Check sheet for the modelled part. Datum: model origin and axes. Units: mm. A direction names the side the tool comes from. Coordinates: 2 decimals unless noted, no trailing zeros. Write each loop counter-clockwise with the first axis right and the second up, starting at its lowest first coordinate (ties: lowest second). Pieces come first, ordered by that corner, then holes. Notation, with made-up numbers: (69, 71) -> (110, 71) arc R12 ccw to (110, 80) -> close; hole circle Ø9 at (79, 0.5). An arc over 180 degrees is marked (long way). One line per item, written item: value. Start each with the question number.
1) Gauge pin test, flat ends, axial feed: P1, Ø2, axis at x = 6.5, y = 8.5, coming from the +Z side; P2, Ø10, axis at x = 12.5, z = -29.5, coming from the -Y side. Record the tip position at first contact, or that the pin passes through.
2) Draft check along Z on faces 1 (the cylindrical face through (-16.76, -3.706, -43.397)), 2 (the cylindrical face through (16.74, 0.11, -37.815)), 3 (the cylindrical face through (-15.846, 12.629, -18.784)). Enter one of: +Z half, -Z half, draft (parallel to the pull), parting line (faces both ways), or undercut.
3) Sectioned sample at A-A on y = 0. Enter the section's corners in (x, z).
4) Sectioned sample at B-B on z = -39.5. Enter the section's corners in (x, y), plus the area to 3 significant figures.
5) Sectioned sample at D-D on x = -5.5. Enter the section's corners in (y, z).
6) Set-up check for faces 4 (the flat face through (-17.5, 4, -33)), 5 (the flat face through (-0.168, 12.845, -18.83)): record each of +Z, -Z, +X, -X, +Y, -Y from which the full face is reachable in a straight line by a thin tool's end or side.
7) Sectioned sample at C-C on z = -34.5. Enter the section's corners in (x, y).
8) Scan lines: line 1 along X through (y, z) = (13, -25); line 2 along Z through (x, y) = (-16.65, 0); line 3 along X through (y, z) = (17.25, -24). Record each from-to range of solid material in increasing order. Write a range as [from, to].
```python
from build123d import *

# Parameters (mm, degrees)
BOSS_EXTRUDE1_DEPTH            = 16
BOSS_EXTRUDE1_DEPTH_BACK       = 16
EDGE_FLANGE1_STRIP_W           = 14
EDGE_FLANGE1_STRIP_H           = 1.5
EDGE_FLANGE1_STRIP_CUT_DEPTH   = 15
EDGE_FLANGE1_STRIP_2_W         = 14
EDGE_FLANGE1_STRIP_2_H         = 1.5
EDGE_FLANGE1_STRIP_CUT_2_DEPTH = 15
EDGE_FLANGE1_DEPTH             = 15
EDGE_FLANGE1_BEND_DEPTH        = 15
CUT_EXTRUDE1_DEPTH             = 70.261521918
CUT_EXTRUDE1_DEPTH_BACK        = 70.261521918
SKETCH12_R                     = 2.5


# Sheet-metal steps are written as plain solids
with BuildPart() as part:
    # Sketch1 → Boss-Extrude1 (new, two sides: drawn at the far end of the back side and taken through both)
    with BuildSketch(Plane(origin=(0, 0, 0), x_dir=(0, 0, -1), z_dir=(1, 0, 0)).offset(-BOSS_EXTRUDE1_DEPTH_BACK)):
        Polygon((13.736581906, 7.002159097), (21.218242798, 20.003110997), (22.518337988, 19.254944908), (15.036677096, 6.253993008), align=None)
    extrude(amount=BOSS_EXTRUDE1_DEPTH + BOSS_EXTRUDE1_DEPTH_BACK)

    # Edge-Flange1 strip (across the edge) → Edge-Flange1 strip cut (cut)
    with BuildSketch(Plane(origin=(16, 19.254944908, -22.518337988), x_dir=(-1, 0, 0), z_dir=(0, -0.8667301266485011, 0.498777392791487))):
        with Locations((-3, -0.75)):
            Rectangle(EDGE_FLANGE1_STRIP_W, EDGE_FLANGE1_STRIP_H)
    extrude(amount=EDGE_FLANGE1_STRIP_CUT_DEPTH, mode=Mode.SUBTRACT)

    # Edge-Flange1 strip 2 (across the edge) → Edge-Flange1 strip cut 2 (cut)
    with BuildSketch(Plane(origin=(-16, 6.253993008, -15.036677096), x_dir=(1, 0, 0), z_dir=(0, 0.8667301266485011, -0.498777392791487))):
        with Locations((-3, -0.75)):
            Rectangle(EDGE_FLANGE1_STRIP_2_W, EDGE_FLANGE1_STRIP_2_H)
    extrude(amount=EDGE_FLANGE1_STRIP_CUT_2_DEPTH, mode=Mode.SUBTRACT)

    # Edge-Flange1 section (across the edge) → Edge-Flange1 (add)
    with BuildSketch(Plane(origin=(16, 19.254944908, -22.518337988), x_dir=(-1, 0, 0), z_dir=(0, -0.8667301266485011, 0.498777392791487))):
        with BuildLine():
            Line((-1.5, 4), (-1.5, 39))
            Line((-1.5, 39), (0, 39))
            Line((0, 39), (0, 4))
            ThreePointArc((0, 4), (1.171572875, 1.171572875), (4, 0))
            Line((4, 0), (4, -1.5))
            ThreePointArc((4, -1.5), (0.110912703, 0.110912703), (-1.5, 4))
        make_face()
    extrude(amount=EDGE_FLANGE1_DEPTH)

    # Edge-Flange1 section 2 (across the edge) → Edge-Flange1 bend (add)
    with BuildSketch(Plane(origin=(-16, 6.253993008, -15.036677096), x_dir=(1, 0, 0), z_dir=(0, 0.8667301266485011, -0.498777392791487))):
        with BuildLine():
            Line((-1.5, 4), (-1.5, 39))
            Line((-1.5, 39), (0, 39))
            Line((0, 39), (0, 4))
            ThreePointArc((0, 4), (1.171572875, 1.171572875), (4, 0))
            Line((4, 0), (4, -1.5))
            ThreePointArc((4, -1.5), (0.110912703, 0.110912703), (-1.5, 4))
        make_face()
    extrude(amount=EDGE_FLANGE1_BEND_DEPTH)

    # Sketch12 → Cut-Extrude1 (cut, two sides: drawn at the far end of the back side and taken through both)
    with BuildSketch(Plane(origin=(17.5, 0, 0), x_dir=(0, 0, -1), z_dir=(1, 0, 0)).offset(-CUT_EXTRUDE1_DEPTH_BACK)):
        with Locations((40.312429407, 0)):
            Circle(SKETCH12_R)
        with BuildLine():
            Line((33.525218207, -4.385612156), (48.839152035, -13.198325311))
            Line((48.839152035, -13.198325311), (56.320812927, -0.197373411))
            Line((56.320812927, -0.197373411), (46.583424145, 5.406204035))
            ThreePointArc((46.583424145, 5.406204035), (43.281589749, -3.793536651), (33.525218207, -4.385612156))
        make_face()
    extrude(amount=CUT_EXTRUDE1_DEPTH + CUT_EXTRUDE1_DEPTH_BACK, mode=Mode.SUBTRACT)


solid = part.part
```
Answers:
1. P1: stops at z = -14.02
1. P2: stops at y = -4.12
2. face 1: parting line
2. face 2: undercut
2. face 3: +Z half
3. outline: (-17.5, -46.19) -> (-16, -46.19) -> (-16, -42.81) -> (-17.5, -42.81) -> close; (-17.5, -37.81) -> (-16, -37.81) -> (-16, -25.9) -> (-17.5, -25.9) -> close; (16, -46.19) -> (17.5, -46.19) -> (17.5, -42.81) -> (16, -42.81) -> close; (16, -37.81) -> (17.5, -37.81) -> (17.5, -25.9) -> (16, -25.9) -> close
4. outline: (-17.5, -5.43) -> (-16, -5.43) -> (-16, -2.36) -> (-17.5, -2.36) -> close; (-17.5, 2.36) -> (-16, 2.36) -> (-16, 9.48) -> (-17.5, 9.48) -> close; (16, -5.43) -> (17.5, -5.43) -> (17.5, -2.36) -> (16, -2.36) -> close; (16, 2.36) -> (17.5, 2.36) -> (17.5, 9.48) -> (16, 9.48) -> close
4. area: 30.6 mm2
5. outline: (6.25, -15.04) -> (19.25, -22.52) -> (20, -21.22) -> (7, -13.74) -> close
6. face 4: +Z, -Z, -X, +Y, -Y
6. face 5: -Z, -Y
7. outline: (-17.5, -4.87) -> (-16, -4.87) -> (-16, 12.36) -> (-17.5, 12.36) -> close; (16, -4.87) -> (17.5, -4.87) -> (17.5, 12.36) -> (16, 12.36) -> close
8. line 1: x = [-17.5, -16], [16, 17.5]
8. line 2: z = [-46.19, -42.81], [-37.81, -25.9]
8. line 3: x = [-17.23, -15.61], [15.61, 17.23]
